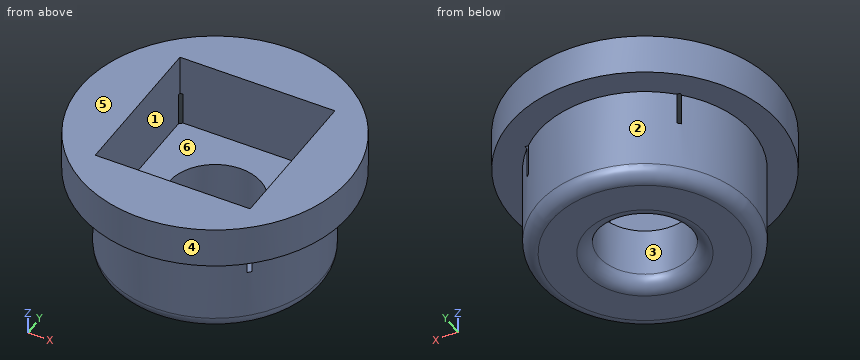
Autodesk Inventor part; units mm, degrees
ref_plane "YZ Plane" through (0, 0, 0) normal (1, 0, 0) x (0, 1, 0)
ref_plane "XZ Plane" through (0, 0, 0) normal (0, 1, 0) x (-1, 0, 0)
ref_plane "XY Plane" through (0, 0, 0) normal (0, 0, 1) x (1, 0, 0)
sketch "Sketch1" plane through (0, 0, 0) normal (1, 0, 0) x (0, 1, 0)
  line L0 (0, 0) -> (1.7, 0) construction
  line L1 (1.7, 0) -> (4.95, 0)
  line L2 (4.95, 0) -> (4.95, -1.5)
  line L3 (4.95, -1.5) -> (3.95, -1.5)
  line L4 (3.95, -1.5) -> (3.95, -5)
  line L5 (3.95, -5) -> (1.7, -5)
  line L6 (1.7, -5) -> (1.7, 0)
  line L7 (0, 0) -> (0, -13.7466) construction
  dimension "d0" = 1.7
  dimension "d1" = 3.95
  dimension "d2" = 1
  dimension "d3" = 1.5
  dimension "d4" = 3.5
revolve "Revolution1" add sketch "Sketch1" angle 360 about axis through (0, 0, 0) along (0, 0, -1)
sketch "Sketch2" plane through (0, 0, 0) normal (0, 0, 1) x (1, 0, 0)
  line L0 (2.85, -2.85) -> (-2.85, -2.85)
  line L1 (-2.85, -2.85) -> (-2.85, 2.85)
  line L2 (-2.85, 2.85) -> (2.85, 2.85)
  line L3 (2.85, 2.85) -> (2.85, -2.85)
  line L4 (2.85, -2.85) -> (-2.85, 2.85) construction
  line L5 (-2.85, -2.85) -> (2.85, 2.85) construction
  point P0 (0, 0)
  dimension "d6" = 5.7
extrude "Extrusion1" cut sketch "Sketch2" against normal blind 2.7
fillet "Fillet1" radius 0.5 2 edges at (0, -3.95, -5) (0, -1.7, -5)
properties part number "HD_BearingShaft1"
Source: CAD feature listing. Evaluate the final solid. Frame: model axes, mm. Face numbers are marked on the shaded views. A direction names the side the tool comes from. Coordinates: 2 decimals unless noted, no trailing zeros. Loops run counter-clockwise (first coordinate to the right, second up) from the corner with the lowest first, then second, coordinate; pieces in that order, holes last. Notation, with made-up numbers: M -35.5,79.5 L -19.5,79.5 A32 cw -19.5,114.5 Z; hole C 64,70.25 d2. An arc over 180 degrees is marked long. Use CSV: the item, a comma, the result in double quotes.
(1) Cut plane A-A on y = 0. Return loops of the section in (x, z), and give its area (3 significant figures).
Answers follow:
outline,"M -4.95,-1.5 L -3.95,-1.5 L -3.95,-4.5 A0.5 ccw -3.45,-5 L -2.2,-5 A0.5 ccw -1.7,-4.5 L -1.7,-2.7 L -2.85,-2.7 L -2.85,0 L -4.95,0 Z; M 1.7,-4.5 A0.5 ccw 2.2,-5 L 3.45,-5 A0.5 ccw 3.95,-4.5 L 3.95,-1.5 L 4.95,-1.5 L 4.95,0 L 2.85,0 L 2.85,-2.7 L 1.7,-2.7 Z"
area,"19.1 mm²"
(2) Reachability of the marked faces 1, 2 and 3 from +Z, -Z, +X, -X, +Y, -Y: full face, straight path, thin tool, end or side. Return the list, or none.
Answers follow:
face 1,"+Z"
face 2,"-Z"
face 3,"+Z, -Z"
(3) Cut plane C-C on z = -1.35. Return loops of the section in (x, y), and give its area (3 significant figures).
Answers follow:
outline,"C 0,0 d9.9; hole M -2.85,-2.85 L 2.85,-2.85 L 2.85,2.85 L -2.85,2.85 Z"
area,"44.5 mm²"
(4) Line query: line 1 (X direction, y = 0, z = -3.3); line 2 (Z direction, x = -4, y = 1). Output: solid intervals per line, ascending. Write a range as [from, to].
Answers follow:
line 1,"[-3.95, -1.7], [1.7, 3.95]"
line 2,"[-1.5, 0]"
(5) Contact query for flat-ended pins moving along their axis: pin 1 (2 mm diameter, centred on y = -1, z = -2, fed in from +X); pin 2 (3 mm diameter, centred on y = -3, z = -4, fed in from -X); pin 3 (2.5 mm diameter, centred on x = 0, y = 0, fed in from -Z); pin 4 (0.8 mm diameter, centred on x = -1.5, z = -1, fed in from -Y). Output: stop coordinate, or through.
Answers follow:
pin 1,"x = 4.95"
pin 2,"x = -3.65"
pin 3,"through"
pin 4,"y = -4.83"
(6) Draft query along X for the marked faces 4, 5 and 6. Return one class per face: pulls with the +X half, pulls with the -X half, needs draft (parallel to the pull), parting line crosses it, or undercut.
Answers follow:
face 4,"parting line crosses it"
face 5,"needs draft"
face 6,"undercut"
(7) Cut plane D-D on y = 4.25. Return loops of the section in (x, z), and give its area (3 significant figures).
Answers follow:
outline,"M -2.54,-1.5 L 2.54,-1.5 L 2.54,0 L -2.54,0 Z"
area,"7.61 mm²"
